Autodesk Inventor part; units mm, degrees
ref_plane "YZ Plane" through (0, 0, 0) normal (1, 0, 0) x (0, 1, 0)
ref_plane "XZ Plane" through (0, 0, 0) normal (0, 1, 0) x (-1, 0, 0)
ref_plane "XY Plane" through (0, 0, 0) normal (0, 0, 1) x (1, 0, 0)
sketch "Sketch1" plane through (0, 0, 0) normal (1, 0, 0) x (0, 1, 0)
  line L0 (-76, 12.5) -> (76, 12.5)
  line L1 (76, 12.5) -> (76, -12.5)
  line L2 (76, -12.5) -> (-76, -12.5)
  line L3 (-76, -12.5) -> (-76, 12.5)
  line L4 (-85.317, 0) -> (85.317, 0) construction
  point P0 (0, 0)
  point P1 (0, 0)
  point P2 (-51, 0)
  point P3 (51, 0)
  dimension "d0" = 152
  dimension "d1" = 25
  dimension "d2" = 76
  dimension "d3" = 12.5
  dimension "d4" = 25
  dimension "d5" = 25
extrude "Extrusion1" add sketch "Sketch1" against normal blind 12
hole "Hole1" at (0, -51, 0) at (0, 51, 0) direction (-1, 0, 0) diameter 9 end through all countersink diameter 17.3 countersink angle 90
properties part number "JAW CAP" material "Steel, Alloy"
Source: CAD feature listing. Evaluate the final solid. Frame: model axes, mm. Coordinates: 2 decimals unless noted, no trailing zeros. Loops run counter-clockwise (first coordinate to the right, second up) from the corner with the lowest first, then second, coordinate; pieces in that order, holes last. Notation, with made-up numbers: (-9.5, 8.5) - (11.5, 8.5) arc R29 cw to (11.5, 40.5) - close; hole circle Ø4 at (13.5, 21). An arc over 180 degrees is marked (long way). One line per item, written item: value. Start each with the question number.
1. Mould query, pull axis Y, two halves, no side actions, for faces 1 (the flat face through (-6, -76, 0)), 2 (the cylindrical face through (-8.13, -46.61, 0.98)), 3 (the flat face through (-6, 76, 0)), 4 (the flat face through (-6, 1, -12.5)). Classes: pulls with the +Y half, pulls with the -Y half, needs draft (parallel to the pull), parting line crosses it, or undercut.
2. Section B-B (x = -9.75). Return the cut outline in (y, z), and give its area (3 significant figures).
3. Section A-A (y = -51). Return the cut outline in (x, z).
4. Contact query for flat-ended pins moving along their axis: P1, Ø1.5, axis at y = 14.5, z = 5.5, coming from the +X side; P2, Ø8, axis at y = -51, z = 0, coming from the -X side. Output: stop coordinate, or through.
5. Section C-C (z = 0). Return the cut outline in (x, y), and give its area (3 significant figures).
6. Ray query, L1, parallel to Y at x = -8.5, z = 0; L2, parallel to Z at x = -6.75, y = -51; L3, parallel to Y at x = -2, z = 1. Return the intervals inside material, ascending.
Verdict:
1. face 1: pulls with the -Y half
1. face 2: undercut
1. face 3: pulls with the +Y half
1. face 4: needs draft
2. outline: (-76, -12.5) - (76, -12.5) - (76, 12.5) - (-76, 12.5) - close; hole circle Ø9 at (-51, 0); hole circle Ø9 at (51, 0)
2. area: 3,670 mm2
3. outline: (-12, -12.5) - (0, -12.5) - (0, -8.65) - (-4.15, -4.5) - (-12, -4.5) - close; (-12, 4.5) - (-4.15, 4.5) - (0, 8.65) - (0, 12.5) - (-12, 12.5) - close
4. P1: stops at x = 0
4. P2: passes through
5. outline: (-12, -76) - (0, -76) - (0, -59.65) - (-4.15, -55.5) - (-12, -55.5) - close; (-12, -46.5) - (-4.15, -46.5) - (0, -42.35) - (0, 42.35) - (-4.15, 46.5) - (-12, 46.5) - close; (-12, 55.5) - (-4.15, 55.5) - (0, 59.65) - (0, 76) - (-12, 76) - close
5. area: 1,570 mm2
6. L1: y = -76 to -55.5, -46.5 to 46.5, 55.5 to 76
6. L2: z = -12.5 to -4.5, 4.5 to 12.5
6. L3: y = -76 to -57.57, -44.43 to 44.43, 57.57 to 76
